Check sheet for the drawn part. Datum: minimum x, y, z corner. Units: mm. A direction names the side the tool comes from. Coordinates: 2 decimals unless noted, no trailing zeros. Write each loop counter-clockwise with the first axis right and the second up, starting at its lowest first coordinate (ties: lowest second). Pieces come first, ordered by that corner, then holes. Notation, with made-up numbers: (16, 82.5) -> (38, 82.5) arc R15 cw to (38, 90.5) -> close; hole circle Ø8 at (75.25, 65). An arc over 180 degrees is marked (long way). Answer in a Markdown table with one row per item.
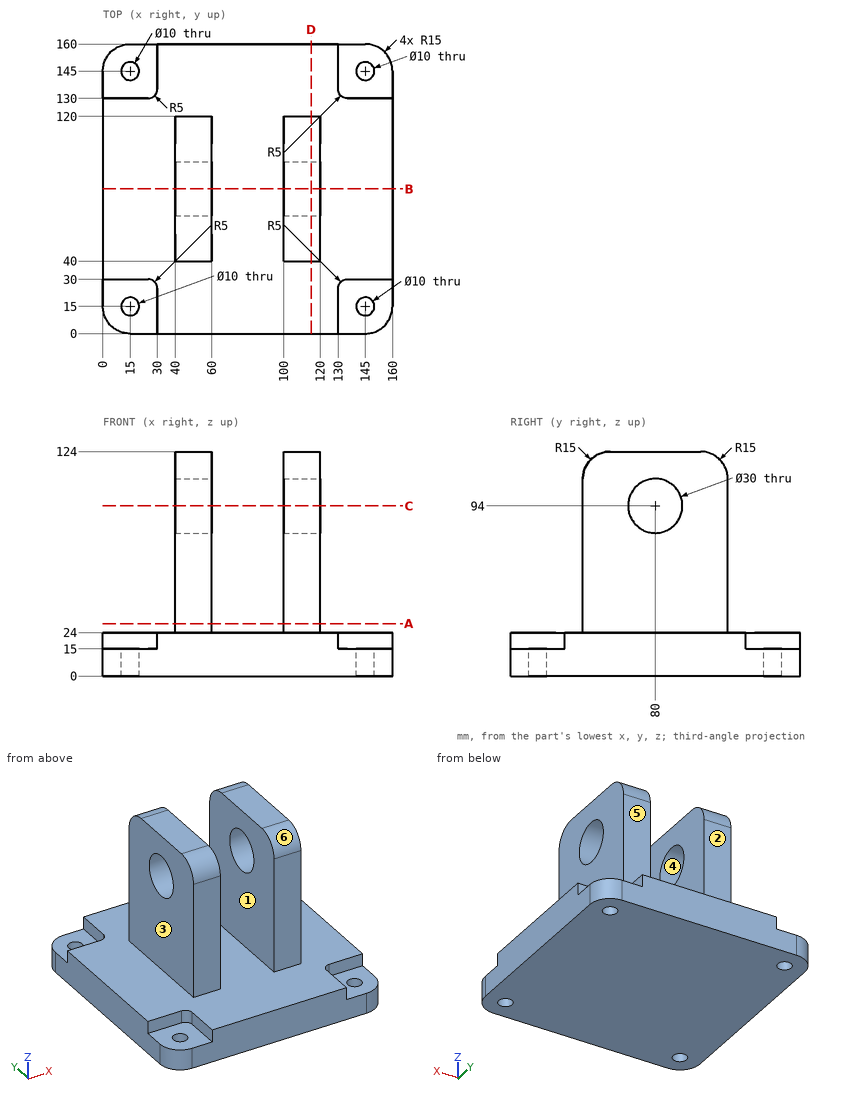
1. Access from +Z, -Z, +X, -X, +Y, -Y to the whole of each face (thin tool, end or side, straight path). Record for the marked faces 1, 2 and 3.
Findings below:
| item | result |
|---|---|
| face 1 | +Z, +Y, -Y |
| face 2 | +Z, +X, -X, +Y |
| face 3 | +Z, -X, +Y, -Y |
2. Sectioned sample at B-B, the plane y = 80. Record the cut outline in (x, z).
Findings below:
| item | result |
|---|---|
| outline | (0, 0) -> (160, 0) -> (160, 24) -> (120, 24) -> (120, 79) -> (100, 79) -> (100, 24) -> (60, 24) -> (60, 79) -> (40, 79) -> (40, 24) -> (0, 24) -> close; (40, 109) -> (60, 109) -> (60, 124) -> (40, 124) -> close; (100, 109) -> (120, 109) -> (120, 124) -> (100, 124) -> close |
3. Sectioned sample at C-C, the plane z = 94. Record the cut outline in (x, y).
Findings below:
| item | result |
|---|---|
| outline | (40, 40) -> (60, 40) -> (60, 65) -> (40, 65) -> close; (40, 95) -> (60, 95) -> (60, 120) -> (40, 120) -> close; (100, 40) -> (120, 40) -> (120, 65) -> (100, 65) -> close; (100, 95) -> (120, 95) -> (120, 120) -> (100, 120) -> close |
4. Go/stop test with flat-tipped pins: pin 1 (8 mm diameter, centred on x = 15, y = 15, fed in from +Z); pin 2 (10 mm diameter, centred on x = 106, z = 51, fed in from -Y); pin 3 (8 mm diameter, centred on x = 64.5, y = 57, fed in from +Z); pin 4 (10 mm diameter, centred on y = 153, z = 19, fed in from -X). Record where each tip stops, or that it passes through.
Findings below:
| item | result |
|---|---|
| pin 1 | passes through |
| pin 2 | stops at y = 40 |
| pin 3 | stops at z = 24 |
| pin 4 | stops at x = 0.86 |
5. Material ranges on probe 1 along Y at (x, z) = (145, 5); probe 2 along Z at (x, y) = (50.75, 80), recorded low to high. Write a range as from..to.
Findings below:
| item | result |
|---|---|
| probe 1 | y = 0..10, 20..140, 150..160 |
| probe 2 | z = 0..79, 109..124 |
6. Release check for a two-part mould opening along Z. For the marked faces 4, 5 and 6 record: released by +Z, released by -Z, zero draft, split by the parting line, or undercut.
Findings below:
| item | result |
|---|---|
| face 4 | undercut |
| face 5 | zero draft |
| face 6 | released by +Z |
7. Sectioned sample at D-D, the plane x = 115. Record the cut outline in (y, z), and give its area (3 significant figures).
Findings below:
| item | result |
|---|---|
| outline | (0, 0) -> (160, 0) -> (160, 24) -> (120, 24) -> (120, 109) arc R15 ccw to (105, 124) -> (55, 124) arc R15 ccw to (40, 109) -> (40, 24) -> (0, 24) -> close; hole circle Ø30 at (80, 94) |
| area | 11,000 mm² |
8. Sectioned sample at A-A, the plane z = 29. Record the cut outline in (x, y), and give its area (3 significant figures).
Findings below:
| item | result |
|---|---|
| outline | (40, 40) -> (60, 40) -> (60, 120) -> (40, 120) -> close; (100, 40) -> (120, 40) -> (120, 120) -> (100, 120) -> close |
| area | 3,200 mm² |
